from build123d import *

# Parameters (mm, degrees)
F0_W     = 30
F0_H     = 60
F0_R     = 5.5
F0_W_2   = 10
F0_H_2   = 2.5
F0_R_2   = 4
F1_DEPTH = 5
F2_DEPTH = 15
F3_W     = 10
F3_H     = 10
F3_R     = 3.6
F4_DEPTH = 15
F5_DEPTH = 25
F6_DEPTH = 10


with BuildPart() as f1:
    # F0 (on Front) → F1 (new body)
    with BuildSketch(Plane.XZ):
        Rectangle(F0_W, F0_H)
        with Locations((0, -20)):
            Circle(F0_R, mode=Mode.SUBTRACT)
        with Locations((0, -6.25)):
            Rectangle(F0_W_2, F0_H_2, mode=Mode.SUBTRACT)
        with Locations((0, 6.25)):
            Rectangle(F0_W_2, F0_H_2, mode=Mode.SUBTRACT)
        with Locations((0, 20)):
            Circle(F0_R, mode=Mode.SUBTRACT)
        with Locations((0, 20)):
            Circle(F0_R)
        with Locations((0, 20)):
            Circle(F0_R_2, mode=Mode.SUBTRACT)
        with Locations((0, -20)):
            Circle(F0_R)
        with Locations((0, -20)):
            Circle(F0_R_2, mode=Mode.SUBTRACT)
    extrude(amount=F1_DEPTH)

    # F0 (on Front) → F2 (join)
    with BuildSketch(Plane.XZ):
        with Locations((0, 20)):
            Circle(F0_R)
        with Locations((0, 20)):
            Circle(F0_R_2, mode=Mode.SUBTRACT)
        with Locations((0, -20)):
            Circle(F0_R)
        with Locations((0, -20)):
            Circle(F0_R_2, mode=Mode.SUBTRACT)
        with Locations((0, 20)):
            Circle(F0_R_2)
        with Locations((0, -20)):
            Circle(F0_R_2)
    extrude(amount=-F2_DEPTH)

    # F3 (on Right) → F4 (join, symmetric)
    with BuildSketch(Plane.YZ):
        with Locations((5, 0)):
            Rectangle(F3_W, F3_H)
        with Locations((4, 0)):
            Circle(F3_R, mode=Mode.SUBTRACT)
        with Locations((4, 0)):
            Circle(F3_R)
    extrude(amount=F4_DEPTH, both=True)

    # F3 (on Right) → F5 (cut, symmetric)
    with BuildSketch(Plane.YZ):
        with Locations((4, 0)):
            Circle(F3_R)
    extrude(amount=F5_DEPTH, both=True, mode=Mode.SUBTRACT)

    # F0 (on Front) → F6 (cut, symmetric)
    with BuildSketch(Plane.XZ):
        with Locations((0, 20)):
            Circle(F0_R_2)
        with Locations((0, -20)):
            Circle(F0_R_2)
    extrude(amount=F6_DEPTH, both=True, mode=Mode.SUBTRACT)


solid = f1.part
Design review of the part built by this model. Coordinates are the model's own, in mm. A direction names the side the tool comes from. Give positions to 0.01 mm unless a question says otherwise; leave off trailing zeros. Loops run counter-clockwise (first coordinate to the right, second up) from the corner with the lowest first, then second, coordinate; pieces in that order, holes last. Notation, with made-up numbers: M 74,11 L 111,11 A28 ccw 111,29 Z; hole C 70,19 d2. An arc over 180 degrees is marked long. One line per question, with ' | ' between items. Start each with the question number.
1. Add section B-B (y = 6). Write out the cut boundary in (x, z), plus the area to 3 significant figures.
2. For faces 5 (the face through (0, 4, -5)), 6 (the face through (0, 10, 0)), 7 (the face through (-5, -2, -6)), list the 3-axis set-ups (+Z, -Z, +X, -X, +Y, -Y) from which the entire face can be reached by the end or side of a thin tool; tool diameter is ignored.
3. To check wall thickness, follow L1, parallel to Z at x = 0, y = -0.5; L2, parallel to Z at x = 2.25, y = 4.5; L3, parallel to Z at x = -3.5, y = 7. State the ranges of each line that lie inside material, in increasing order.
4. Add section D-D (x = -7.5). Write out the cut boundary in (y, z), plus the area to 3 significant figures.
5. Add section A-A (x = 0). Give the number of separate pieces and of enclosed holes in the cut face, plus the area to 3 significant figures.
6. The part is to be moulded in two halves that separate along X. For faces 1 (the face through (-4.05, 7.4, -16.28)), 2 (the face through (-0.521, 2.605, -16.034)), 3 (the face through (0, -2, 7.5)), 4 (the face through (0, -2, 30)), say which applies: released by +X, released by -X, zero draft, split by the parting line, or undercut.
7. Add section C-C (z = 0). Write out the cut boundary in (x, y).
8. Insertion check: P1, Ø8, axis at x = -4.5, z = -0.5, coming from the +Y side; P2, Ø2, axis at x = -12, y = 6.5, coming from the -Z side; P3, Ø1, axis at y = 7.5, z = -14.5, coming from the +X side. Each pin has a flat end and moves straight along its axis. Give the tip position at first contact, or say it passes through.
Worked out:
1) outline: M -15,-5 L 15,-5 L 15,-2.99 L -15,-2.99 Z; M -15,2.99 L 15,2.99 L 15,5 L -15,5 Z; C 0,-20 d11; C 0,20 d11; hole C 0,-20 d8; hole C 0,20 d8 | area: 210 mm²
2) face 5: +Y | face 6: +X, -X, +Y | face 7: +Y, -Y
3) L1: z = -30 to -24, -16 to -7.5, -5 to 5, 7.5 to 16, 24 to 30 | L2: z = -25.02 to -23.31, -16.69 to -14.98, -5 to -3.57, 3.57 to 5, 14.98 to 16.69, 23.31 to 25.02 | L3: z = -24.24 to -21.94, -18.06 to -15.76, -5 to -1.99, 1.99 to 5, 15.76 to 18.06, 21.94 to 24.24
4) outline: M -5,-30 L 0,-30 L 0,-5 L 10,-5 L 10,5 L 0,5 L 0,30 L -5,30 Z; hole C 4,0 d7.2 | area: 359 mm²
5) separate pieces: 3 | enclosed holes: 1 | area: 424 mm²
6) face 1: split by the parting line | face 2: undercut | face 3: undercut | face 4: zero draft
7) outline: M -15,-5 L 15,-5 L 15,0.4 L -15,0.4 Z; M -15,7.6 L 15,7.6 L 15,10 L -15,10 Z
8) P1: stops at y = 10 | P2: stops at z = -5 | P3: stops at x = 2.29
